Autodesk Inventor part; units mm, degrees
ref_plane "YZ Plane" through (0, 0, 0) normal (1, 0, 0) x (0, 1, 0)
ref_plane "XZ Plane" through (0, 0, 0) normal (0, 1, 0) x (-1, 0, 0)
ref_plane "XY Plane" through (0, 0, 0) normal (0, 0, 1) x (1, 0, 0)
sketch "Sketch1" plane through (0, 0, 0) normal (0, 1, 0) x (-1, 0, 0)
  arc A0 (-4.5826, -2) -> (0, -5) centre (0, 0) ccw
  line L0 (47.5826, -2) -> (24.5826, -2)
  arc A1 (20, -5) -> (24.5826, -2) centre (20, 0) ccw
  line L1 (0, -5) -> (20, -5)
  line L2 (49.5826, 0) -> (49.5826, 6)
  line L3 (47.5826, 8) -> (24.5826, 8)
  arc A2 (49.5826, 6) -> (47.5826, 8) centre (47.5826, 6) ccw
  arc A3 (47.5826, -2) -> (49.5826, 0) centre (47.5826, 0) ccw
  line L4 (-4.5826, -2) -> (-27.5826, -2)
  line L5 (-29.5826, 0) -> (-29.5826, 6)
  line L6 (-27.5826, 8) -> (-4.5826, 8)
  line L7 (24.5826, 8) -> (24.5826, 21)
  line L8 (24.5826, 21) -> (-4.5826, 21)
  line L9 (-4.5826, 21) -> (-4.5826, 8)
  arc A4 (-29.5826, 0) -> (-27.5826, -2) centre (-27.5826, 0) ccw
  arc A5 (-27.5826, 8) -> (-29.5826, 6) centre (-27.5826, 6) ccw
  point P0 (49.5826, -2)
  point P1 (49.5826, 8)
  point P2 (-29.5826, -2)
  point P3 (-29.5826, 8)
  dimension "d0" = 5
  dimension "d8" = 5
  dimension "d9" = 20
  dimension "d12" = 3
  dimension "d14" = 10
  dimension "d15" = 2
  dimension "d49" = 25
  dimension "d50" = 25
  dimension "d51" = 10
  dimension "d52" = 26
  dimension "d53" = 2
extrude "Extrusion1" add sketch "Sketch1" along normal blind 7
fillet "Fillet2" radius 5 2 edges at (-24.5826, 3.5, 21) (4.5826, 3.5, 21)
sketch "Sketch7" plane through (-24.5826, 0, -2) normal (0, 0, -1) x (-1, 0, 0)
  line L0 (0, 7) -> (23, 7)
  line L1 (-52.1652, 0) -> (-29.1652, 0)
  line L2 (-29.1652, 0) -> (-29.1652, 7)
  line L3 (-52.1652, 7) -> (-29.1652, 7)
  line L4 (-52.1652, 0) -> (-52.1652, 7)
  line L5 (-51.5652, 1.75) -> (-29.1652, 1.75)
  line L6 (-29.1652, 1.75) -> (-29.1652, 5.25)
  line L7 (-29.1652, 5.25) -> (-51.5652, 5.25)
  line L8 (-51.5652, 5.25) -> (-51.5652, 1.75)
  line L9 (0, 1.75) -> (22.4, 1.75)
  line L10 (22.4, 1.75) -> (22.4, 5.25)
  line L11 (22.4, 5.25) -> (0, 5.25)
  line L12 (0, 5.25) -> (0, 1.75)
  line L13 (-54.1652, 0) -> (-54.1652, 7)
  line L14 (25, 0) -> (25, 7)
  point P0 (-24.5826, 0)
  dimension "d55" = 22.4
  dimension "d56" = 3.5
  dimension "d57" = 1.75
  dimension "d58" = 2.6
  dimension "d59" = 2.6
extrude "Extrusion7" cut sketch "Sketch7" against normal up to next contours L5 L8 L7 L2 | L12 L11 L10 L9
sketch "Sketch8" plane through (0, 0, 0) normal (0, -1, 0) x (1, 0, 0)
  line L0 (-24.5826, 8) -> (-24.5826, 16)
  line L1 (0, -5) -> (-20, -5)
  circle A0 centre (-10.0001, 7) radius 9
  circle A1 centre (-10.0001, 7) radius 7
  dimension "d62" = 18
  dimension "d63" = 12
  dimension "d64" = 14
  dimension "d65" = 14.5825
extrude "Extrusion8" cut sketch "Sketch8" against normal blind 5
sketch "Sketch11" plane through (0, 7, 0) normal (0, 1, 0) x (1, 0, 0)
  arc A0 (4.5826, 2) -> (0, 5) centre (0, 0) ccw
  line L0 (0, 5) -> (-20, 5)
  arc A1 (-20, 5) -> (-24.5826, 2) centre (-20, 0) ccw
  line L1 (-24.5826, 2) -> (-47.5826, 2)
  line L2 (4.5826, 2) -> (-24.5826, 2)
extrude "Extrusion11" add sketch "Sketch11" along normal blind 5.5
fillet "Fillet3" radius 1 4 edges at (-22.7386, 12.5, -4.1833) (2.7386, 12.5, -4.1833) (-10, 12.5, -5) (-10, 12.5, -2)
sketch "Sketch12" plane through (0, 7, 0) normal (0, 1, 0) x (1, 0, 0)
  circle A0 centre (-10.0001, -7) radius 7
  point P0 (0, 0)
hole "Hole1" at (-10.0001, 7, 7) direction (0, -1, 0) diameter 4 end through all counterbore diameter 7.4 counterbore depth 4.5
properties part number "BedClipUltiBotsMiddle" material "ABS Plastic"
Input: part model. Units: mm. Frame: model coordinates. A direction names the side the tool comes from. Give positions to 0.01 mm unless a question says otherwise; leave off trailing zeros. Order: outer loops, then holes, each group sorted by start corner. A loop starts at its lowest first (then second) coordinate and runs counter-clockwise, first axis right, second up. Notation, with made-up numbers: M 36,51.5 L 56,51.5 A12 cw 56,57.5 Z; hole C 39.5,69 d4. An arc over 180 degrees is marked long. Return JSON: item names as keys, results as strings.
Item 1: Cut plane B-B (z = 7). Return loops of the section in (x, y), then the cut area to 3 significant figures.
Solutions:
{"outline": "M -49.31,0 L -19,0 L -19,5 L -17,5 L -17,0 L -12,0 L -12,2.5 L -13.7,2.5 L -13.7,7 L -49.31,7 Z; M -8,0 L -3,0 L -3,5 L -1,5 L -1,0 L 29.31,0 L 29.31,7 L -6.3,7 L -6.3,2.5 L -8,2.5 Z; hole M -46.98,1.75 L -24.58,1.75 L -24.58,5.25 L -46.98,5.25 Z; hole M 4.58,1.75 L 26.98,1.75 L 26.98,5.25 L 4.58,5.25 Z", "area": "330 mm^2"}
Item 2: Cut plane D-D (z = 11.75). Return loops of the section in (x, y).
Solutions:
{"outline": "M -24.58,0 L -17.64,0 L -17.64,5 L -15.14,5 L -15.14,0 L -4.86,0 L -4.86,5 L -2.36,5 L -2.36,0 L 4.58,0 L 4.58,7 L -24.58,7 Z"}
Item 3: Pull-direction query (Y, two-part tool) for faces 6 (the flat face through (-8, 0, 6)), 7 (the flat face through (4.583, 3, 9)), 8 (the cylindrical face through (3, 6, -4)); classes: +Y half, -Y half, draft (parallel to the pull), parting line (faces both ways), or undercut.
Solutions:
{"face 6": "-Y half", "face 7": "undercut", "face 8": "draft"}
Item 4: Cut plane C-C (y = 8). Return loops of the section in (x, z).
Solutions:
{"outline": "M -24.58,-2 A5 ccw -20,-5 L 0,-5 A5 ccw 4.58,-2 Z"}
Item 5: Access query for faces 1 (the flat face through (16, 1, -2)), 2 (the cylindrical face through (-11.518, 2.465, 0.166)), 3 (the flat face through (-46.983, 3, 3)), 4 (the flat face through (-24.583, 3, 9)), 5 (the flat face through (-8, 2.5, 9)). Directions: +Z, -Z, +X, -X, +Y, -Y. A direction counts if a zero-diameter tool reaches every point of the face in a straight line with its end or side. Return the directions, or none.
Solutions:
{"face 1": "-Z, +X, +Y, -Y", "face 2": "-Y", "face 3": "+Z, -Z", "face 4": "+Z", "face 5": "+Y"}
Item 6: Cut plane A-A (x = -36.5). Return loops of the section in (y, z).
Solutions:
{"outline": "M 0,-2 L 1.75,-2 L 1.75,8 L 0,8 Z; M 5.25,-2 L 7,-2 L 7,8 L 5.25,8 Z"}
Item 7: First-contact query: P1, Ø3.5, axis at x = -10, z = 6, coming from the +Y side; P2, Ø1.3, axis at x = -16.5, y = 9.5, coming from the +Z side; P3, Ø1.5, axis at y = 6, z = -1.5, coming from the -X side; P4, Ø2, axis at y = 11, z = 0.5, coming from the -X side. Flat tips, straight axial feed; report the tip coordinate or a pass-through.
Solutions:
{"P1": "y = 2.5", "P2": "z = -2", "P3": "x = -49.44", "P4": "through"}
Item 8: Ray query, probe 1 along X at (y, z) = (4.5, 11); probe 2 along X at (y, z) = (5.1, 7); probe 3 along Y at (x, z) = (-34.5, 1.75). Return the intervals inside material, ascending.
Solutions:
{"probe 1": "-24.58 to -18.06, -15.74 to -4.26, -1.94 to 4.58", "probe 2": "-49.31 to -46.98, -24.58 to -13.7, -6.3 to 4.58, 26.98 to 29.31", "probe 3": "0 to 1.75, 5.25 to 7"}
